Source: CAD feature listing. Evaluate the final solid. Frame: model axes, mm. A direction names the side the tool comes from. Give positions to 0.01 mm unless a question says otherwise; leave off trailing zeros. Order: outer loops, then holes, each group sorted by start corner. A loop starts at its lowest first (then second) coordinate and runs counter-clockwise, first axis right, second up. Notation, with made-up numbers: (65.25, -32) -> (114.25, -32) arc R5 cw to (114.25, -24) -> close; hole circle Ø5 at (75, 9). An arc over 180 degrees is marked (long way). Use CSV: the item, a comma, the result in double quotes.
```python
from build123d import *

# Parameters (mm, degrees)
F0_R       = 4.5
F1_DEPTH   = 8
F2_SIZE2   = 0.6
F2_SIZE    = 2
F2_2_SIZE2 = 0.6
F2_2_SIZE  = 2
F3_DEPTH   = 1.5


# Not quite as in the source:
# - a feature names something its author has since deleted; it is built from what else it names


with BuildPart() as f1:
    # F0 (on Top) → F1 (new body)
    with BuildSketch(Plane.XY):
        Circle(F0_R)
        with BuildLine():
            ThreePointArc((3.2496153619, 1), (3.3621936463, 0.5056222749), (3.4, 0))
            ThreePointArc((3.4, 0), (3.3621936463, -0.5056222749), (3.2496153619, -1))
            ThreePointArc((3.2496153619, -1), (0, -3.4), (-3.2496153619, -1))
            ThreePointArc((-3.2496153619, -1), (-3.4, 0), (-3.2496153619, 1))
            ThreePointArc((-3.2496153619, 1), (0, 3.4), (3.2496153619, 1))
        make_face(mode=Mode.SUBTRACT)
        with BuildLine():
            ThreePointArc((3.2496153619, -1), (3.3621936463, -0.5056222749), (3.4, 0))
            ThreePointArc((3.4, 0), (3.3621936463, 0.5056222749), (3.2496153619, 1))
            Line((3.2496153619, 1), (-3.2496153619, 1))
            ThreePointArc((-3.2496153619, 1), (-3.4, 0), (-3.2496153619, -1))
            Line((-3.2496153619, -1), (3.2496153619, -1))
        make_face()
    extrude(amount=F1_DEPTH)

    # F2
    f2_edges = [f1.edges().sort_by_distance(p)[0] for p in [
        (0, 1, 8),
    ]]
    f2_side = f1.faces().sort_by_distance((0, 1, 4))[0]
    chamfer(f2_edges, length=F2_SIZE, length2=F2_SIZE2, reference=f2_side)

    # F2#2
    f2_2_edges = [f1.edges().sort_by_distance(p)[0] for p in [
        (0, -1, 8),
    ]]
    f2_2_side = f1.faces().sort_by_distance((0, -1, 4))[0]
    chamfer(f2_2_edges, length=F2_2_SIZE, length2=F2_2_SIZE2, reference=f2_2_side)

    # F0 (on Top) → F3 (join)
    with BuildSketch(Plane.XY):
        Circle(F0_R)
        with BuildLine():
            ThreePointArc((3.2496153619, 1), (3.3621936463, 0.5056222749), (3.4, 0))
            ThreePointArc((3.4, 0), (3.3621936463, -0.5056222749), (3.2496153619, -1))
            ThreePointArc((3.2496153619, -1), (0, -3.4), (-3.2496153619, -1))
            ThreePointArc((-3.2496153619, -1), (-3.4, 0), (-3.2496153619, 1))
            ThreePointArc((-3.2496153619, 1), (0, 3.4), (3.2496153619, 1))
        make_face(mode=Mode.SUBTRACT)
        with BuildLine():
            ThreePointArc((3.2496153619, -1), (3.3621936463, -0.5056222749), (3.4, 0))
            ThreePointArc((3.4, 0), (3.3621936463, 0.5056222749), (3.2496153619, 1))
            Line((3.2496153619, 1), (-3.2496153619, 1))
            ThreePointArc((-3.2496153619, 1), (-3.4, 0), (-3.2496153619, -1))
            Line((-3.2496153619, -1), (3.2496153619, -1))
        make_face()
        with BuildLine():
            Line((-3.2496153619, 1), (3.2496153619, 1))
            ThreePointArc((3.2496153619, 1), (0, 3.4), (-3.2496153619, 1))
        make_face()
        with BuildLine():
            ThreePointArc((-3.2496153619, -1), (0, -3.4), (3.2496153619, -1))
            Line((3.2496153619, -1), (-3.2496153619, -1))
        make_face()
    extrude(amount=-F3_DEPTH)


solid = f1.part
```
1. Ray query, line 1 along Y through (x, z) = (0.75, 2.25); line 2 along Y through (x, z) = (0.5, 2.75); line 3 along Z through (x, y) = (-1, 1.5). Return the intervals inside material, ascending.
Answer below:
line 1,"y = -4.44 to -3.32, -1 to 1, 3.32 to 4.44"
line 2,"y = -4.47 to -3.36, -1 to 1, 3.36 to 4.47"
line 3,"z = -1.5 to 0"
2. Section query A-A on z = 3.25. Return loops of the section in (x, y), plus the area to 3 significant figures.
Answer below:
outline,"circle Ø9 at (0, 0); hole (-3.25, -1) arc R3.4 ccw to (3.25, -1) -> close; hole (-3.25, 1) -> (3.25, 1) arc R3.4 ccw to start"
area,"40.7 mm²"
3. Section query B-B on x = 0. Return loops of the section in (y, z).
Answer below:
outline,"(-4.5, -1.5) -> (4.5, -1.5) -> (4.5, 8) -> (3.4, 8) -> (3.4, 0) -> (1, 0) -> (1, 6) -> (0.4, 8) -> (-0.4, 8) -> (-1, 6) -> (-1, 0) -> (-3.4, 0) -> (-3.4, 8) -> (-4.5, 8) -> close"
4. Pin query (flat end, axial travel): P1, Ø3, axis at x = -1, z = 3.5, coming from the -Y side; P2, Ø4, axis at x = -2.5, z = 0.5, coming from the +Y side; P3, Ø1.9, axis at x = 0, y = -2, coming from the +Z side. Return the tip coordinate at first contact, or that it passes through.
Answer below:
P1,"stops at y = -4.5"
P2,"stops at y = 4.47"
P3,"stops at z = 0"
5. Section query C-C on y = -2.5. Return loops of the section in (x, z).
Answer below:
outline,"(-3.74, -1.5) -> (3.74, -1.5) -> (3.74, 8) -> (2.3, 8) -> (2.3, 0) -> (-2.3, 0) -> (-2.3, 8) -> (-3.74, 8) -> close"
6. Access query for faces 4 (the flat face through (0, -2, 0)), 5 (the flat face through (0, 0, 8)). Directions: +Z, -Z, +X, -X, +Y, -Y. A direction counts if a zero-diameter tool reaches every point of the face in a straight line with its end or side. Return the directions, or none.
Answer below:
face 4,"+Z"
face 5,"+Z, +X, -X, +Y, -Y"
7. Section query D-D on z = -0.25. Return loops of the section in (x, y), plus the area to 3 significant figures.
Answer below:
outline,"circle Ø9 at (0, 0)"
area,"63.6 mm²"
8. Mould query, pull axis X, two halves, no side actions, for faces 1 (the flat face through (0, 0, -1.5)), 2 (the cylindrical face through (-0.59, 4.46, 3.32)), 3 (the flat face through (0, 2, 0)). Classes: released by +X, released by -X, zero draft, split by the parting line, or undercut.
Answer below:
face 1,"zero draft"
face 2,"split by the parting line"
face 3,"undercut"
